Verification items for the finished model (mm, model axes). Face numbers are marked on the shaded views. A direction names the side the tool comes from. Coordinates: 2 decimals unless noted, no trailing zeros. Write each loop counter-clockwise with the first axis right and the second up, starting at its lowest first coordinate (ties: lowest second). Pieces come first, ordered by that corner, then holes. Notation, with made-up numbers: (19, 38.5) -> (37, 38.5) arc R19 cw to (37, 47.5) -> close; hole circle Ø3 at (21, 60). An arc over 180 degrees is marked (long way). Use CSV: the item, a comma, the result in double quotes.
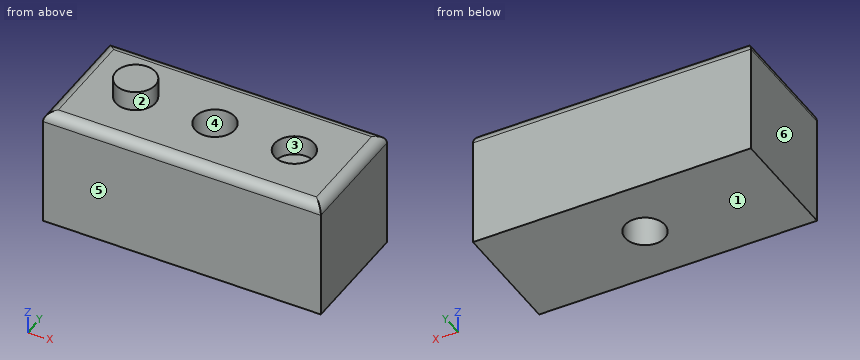
```python
from build123d import *

# Parameters (mm, degrees)
F0_W     = 140
F0_H     = 60
F1_DEPTH = 60
F2_R     = 10
F5_DEPTH = 10
F3_R     = 10
F6_DEPTH = 10
F4_R     = 10
F7_DEPTH = 109.5
F8_R     = 5


with BuildPart() as f1:
    # F0 (on Top) → F1 (new body)
    with BuildSketch(Plane.XY):
        Rectangle(F0_W, F0_H)
    extrude(amount=F1_DEPTH)

    # F2 (on face) → F5 (join)
    with BuildSketch(Plane.XY.offset(60)):
        with Locations((-40, 0)):
            Circle(F2_R)
    extrude(amount=F5_DEPTH)

    # F3 (on face) → F6 (cut)
    with BuildSketch(Plane.XY.offset(60)):
        with Locations((40, 0)):
            Circle(F3_R)
    extrude(amount=-F6_DEPTH, mode=Mode.SUBTRACT)

    # F4 (on face) → F7 (cut)
    with BuildSketch(Plane.XY.offset(60)):
        Circle(F4_R)
    extrude(amount=-F7_DEPTH, mode=Mode.SUBTRACT)

    # F8
    f8_edges = [f1.edges().sort_by_distance(p)[0] for p in [
        (-70, 0, 60),
        (0, 30, 60),
        (70, 0, 60),
        (0, -30, 60),
    ]]
    fillet(f8_edges, radius=F8_R)


solid = f1.part
```
1) Scan lines: L1, parallel to Y at x = 40, z = 52.5; L2, parallel to Z at x = -62.5, y = 20.5; L3, parallel to X at y = 7.5, z = 56.5. Record each from-to range of solid material in increasing order.
Return value:
L1,"-30 to -10, 10 to 30"
L2,"0 to 60"
L3,"-69.77 to -6.61, 6.61 to 33.39, 46.61 to 69.77"
2) Cross-section at C-C (z = 53.5). Record the boundary of the cut face in (x, y), plus the area to 3 significant figures.
Return value:
outline,"(-70, -30) -> (70, -30) -> (70, 30) -> (-70, 30) -> close; hole circle Ø20 at (0, 0); hole circle Ø20 at (40, 0)"
area,"7,770 mm2"
3) Cross-section at B-B (x = -6). Record the boundary of the cut face in (y, z), plus the area to 3 significant figures.
Return value:
outline,"(-30, 0) -> (-8, 0) -> (-8, 60) -> (-25, 60) arc R5 ccw to (-30, 55) -> close; (8, 0) -> (30, 0) -> (30, 55) arc R5 ccw to (25, 60) -> (8, 60) -> close"
area,"2,630 mm2"
4) Set-up check for the marked faces 1 and 2: record each of +Z, -Z, +X, -X, +Y, -Y from which the full face is reachable in a straight line by a thin tool's end or side.
Return value:
face 1,"-Z, +X, -X, +Y, -Y"
face 2,"+Z"
5) Mould release check, pull along X, two halves, no side actions. Record for the marked faces 3, 4, 5 and 6: released by +X, released by -X, zero draft, split by the parting line, or undercut.
Return value:
face 3,"undercut"
face 4,"undercut"
face 5,"zero draft"
face 6,"released by -X"
6) Cross-section at D-D (z = 21.5). Record the boundary of the cut face in (x, y).
Return value:
outline,"(-70, -30) -> (70, -30) -> (70, 30) -> (-70, 30) -> close; hole circle Ø20 at (0, 0)"
7) Cross-section at A-A (y = 0). Record the boundary of the cut face in (x, z).
Return value:
outline,"(-70, 0) -> (-10, 0) -> (-10, 60) -> (-30, 60) -> (-30, 70) -> (-50, 70) -> (-50, 60) -> (-65, 60) arc R5 ccw to (-70, 55) -> close; (10, 0) -> (70, 0) -> (70, 55) arc R5 ccw to (65, 60) -> (50, 60) -> (50, 50) -> (30, 50) -> (30, 60) -> (10, 60) -> close"
8) Gauge pin test, flat ends, axial feed: pin 1 (10 mm diameter, centred on x = -7, z = 61.5, fed in from +Y); pin 2 (12 mm diameter, centred on x = 29.5, y = 7, fed in from +Z); pin 3 (18 mm diameter, centred on x = 40, y = 0, fed in from +Z). Record the tip position at first contact, or that the pin passes through.
Return value:
pin 1,"y = 29.77"
pin 2,"z = 60"
pin 3,"z = 50"
